from build123d import *

# Parameters (mm, degrees)
SKETCH1_W           = 203.2
SKETCH1_H           = 120.65
BOSS_EXTRUDE1_DEPTH = 50.8
SKETCH2_W           = 196.85
SKETCH2_H           = 114.3
CUT_EXTRUDE1_DEPTH  = 51.8
SKETCH4_W           = 203.2
SKETCH4_H           = 120.65
SKETCH4_W_2         = 196.85
SKETCH4_H_2         = 114.3
BOSS_EXTRUDE2_DEPTH = 6.35
CUT_EXTRUDE5_DEPTH  = 121.65
CUT_EXTRUDE6_REACH  = 205.2
CUT_EXTRUDE7_REACH  = 205.2
SKETCH13_R          = 12.55395
CUT_EXTRUDE8_DEPTH  = 51.8


with BuildPart() as part:
    # Sketch1 → Boss-Extrude1 (new body)
    with BuildSketch(Plane(origin=(0, 0, 0), x_dir=(1, 0, 0), z_dir=(0, 1, 0))):
        Rectangle(SKETCH1_W, SKETCH1_H)
    extrude(amount=BOSS_EXTRUDE1_DEPTH)

    # Sketch2 → Cut-Extrude1 (cut, through all)
    with BuildSketch(Plane(origin=(0, 50.8, 0), x_dir=(1, 0, 0), z_dir=(0, 1, 0))):
        Rectangle(SKETCH2_W, SKETCH2_H)
    extrude(amount=-CUT_EXTRUDE1_DEPTH, mode=Mode.SUBTRACT)

    # Sketch4 → Boss-Extrude2 (add)
    with BuildSketch(Plane(origin=(0, 50.8, 0), x_dir=(1, 0, 0), z_dir=(0, 1, 0))):
        Rectangle(SKETCH4_W, SKETCH4_H)
        Rectangle(SKETCH4_W_2, SKETCH4_H_2, mode=Mode.SUBTRACT)
    extrude(amount=-BOSS_EXTRUDE2_DEPTH)

    # Sketch10 → Cut-Extrude5 (cut, through all)
    with BuildSketch(Plane.XY.offset(60.325)):
        with BuildLine():
            ThreePointArc((-65.9511, 22.225), (-81.206975571, 31.167602912), (-81.556705839, 13.4874))
            Line((-81.556705839, 13.4874), (-70.843294161, 13.4874))
            ThreePointArc((-70.843294161, 13.4874), (-67.257397088, 17.218024429), (-65.9511, 22.225))
        make_face()
        with BuildLine():
            ThreePointArc((-15.1511, 22.225), (-30.406975571, 31.167602912), (-30.756705839, 13.4874))
            Line((-30.756705839, 13.4874), (-20.043294161, 13.4874))
            ThreePointArc((-20.043294161, 13.4874), (-16.457397088, 17.218024429), (-15.1511, 22.225))
        make_face()
        with BuildLine():
            ThreePointArc((35.6489, 22.225), (20.393024429, 31.167602912), (20.043294161, 13.4874))
            Line((20.043294161, 13.4874), (30.756705839, 13.4874))
            ThreePointArc((30.756705839, 13.4874), (34.342602912, 17.218024429), (35.6489, 22.225))
        make_face()
        with BuildLine():
            Line((70.843294161, 13.4874), (81.556705839, 13.4874))
            ThreePointArc((81.556705839, 13.4874), (85.142602912, 17.218024429), (86.4489, 22.225))
            ThreePointArc((86.4489, 22.225), (71.193024429, 31.167602912), (70.843294161, 13.4874))
        make_face()
    extrude(amount=-CUT_EXTRUDE5_DEPTH, mode=Mode.SUBTRACT)

    # Sketch12 → Cut-Extrude6 (cut, up to next)
    with BuildSketch(Plane(origin=(101.6, 0, 0), x_dir=(0, 0, -1), z_dir=(1, 0, 0)), mode=Mode.PRIVATE) as cut_extrude6_sk1:
        with BuildLine():
            ThreePointArc((-16.868294161, 13.4874), (-22.225, 32.4739), (-27.581705839, 13.4874))
            Line((-27.581705839, 13.4874), (-16.868294161, 13.4874))
        make_face()
    cut_extrude6_tool1 = extrude(cut_extrude6_sk1.sketch, amount=-CUT_EXTRUDE6_REACH, mode=Mode.PRIVATE) & part.part
    add(cut_extrude6_tool1.solids().sort_by_distance((101.6, 22.546198, 22.225))[0], mode=Mode.SUBTRACT)
    # Sketch12 → Cut-Extrude6 (cut, up to next)
    with BuildSketch(Plane(origin=(101.6, 0, 0), x_dir=(0, 0, -1), z_dir=(1, 0, 0)), mode=Mode.PRIVATE) as cut_extrude6_sk2:
        with BuildLine():
            ThreePointArc((27.581705839, 13.4874), (22.225, 32.4739), (16.868294161, 13.4874))
            Line((16.868294161, 13.4874), (27.581705839, 13.4874))
        make_face()
    cut_extrude6_tool2 = extrude(cut_extrude6_sk2.sketch, amount=-CUT_EXTRUDE6_REACH, mode=Mode.PRIVATE) & part.part
    add(cut_extrude6_tool2.solids().sort_by_distance((101.6, 22.546198, -22.225))[0], mode=Mode.SUBTRACT)

    # Sketch13 → Cut-Extrude7 (cut, up to next)
    with BuildSketch(Plane.ZY.offset(101.6), mode=Mode.PRIVATE) as cut_extrude7_sk1:
        with Locations((12.7, 28.575)):
            Circle(SKETCH13_R)
    cut_extrude7_tool1 = extrude(cut_extrude7_sk1.sketch, amount=-CUT_EXTRUDE7_REACH, mode=Mode.PRIVATE) & part.part
    add(cut_extrude7_tool1.solids().sort_by_distance((-101.6, 28.575, 12.7))[0], mode=Mode.SUBTRACT)

    # Sketch14 → Cut-Extrude8 (cut, through all)
    with BuildSketch(Plane(origin=(0, 50.8, 0), x_dir=(1, 0, 0), z_dir=(0, 1, 0))):
        Polygon((-98.425, -57.15), (-98.425, -60.325), (101.6, -60.325), (101.6, 60.325), (-98.425, 60.325), align=None)
    extrude(amount=-CUT_EXTRUDE8_DEPTH, mode=Mode.SUBTRACT)


solid = part.part
For this review, take the finished solid that the model builds, in its own axes (mm). Round coordinates to 2 decimals unless told otherwise and drop trailing zeros. Write each loop counter-clockwise with the first axis right and the second up, starting at its lowest first coordinate (ties: lowest second). Pieces come first, ordered by that corner, then holes. Notation, with made-up numbers: M 33.25,32 L 83.25,32 A19 ccw 83.25,67 Z; hole C 2,17.5 d3. An arc over 180 degrees is marked long. Write item = value, one per line. Start each with the question number.
(1) We need section A-A (z = 24). Give the boundary of the cut face in (x, y) (3 decimals), then the cut area to 3 significant figures.
(2) We need section C-C (y = 31.5). Give the boundary of the cut face in (x, z) (3 decimals), then the cut area to 3 significant figures.
(3) We need section B-B (x = -100.55). Give the boundary of the cut face in (y, z) (3 decimals).
(4) For line 1 along Y through (x, z) = (-99.6, 12.7); line 2 along Z through (x, y) = (-99.1, 25) (3 decimals); line 3 along Z through (x, y) = (-100.35, 20) (3 decimals), list the stretches that pass through material, from the lowest coordinate up.
(5) The part is to be moulded in two halves that separate along Y. For faces 1 (the face through (-100, 50.8, -1)), 2 (the face through (-100, 25, -60.325)), 3 (the face through (-100.03, 37.06, 3.45)), say which applies: +Y half, -Y half, draft (parallel to the pull), parting line (faces both ways), or undercut.
Results found:
q1.outline = M -101.6,0 L -98.425,0 L -98.425,23.106 L -101.6,23.106 Z; M -101.6,34.044 L -98.425,34.044 L -98.425,50.8 L -101.6,50.8 Z
q1.area = 127 mm²
q2.outline = M -101.6,-60.325 L -98.425,-60.325 L -98.425,0.492 L -101.6,0.492 Z; M -101.6,24.908 L -98.425,24.908 L -98.425,60.325 L -101.6,60.325 Z
q2.area = 306 mm²
q3.outline = M 0,-60.325 L 50.8,-60.325 L 50.8,60.325 L 0,60.325 Z; hole C 28.575,12.7 d25.108
q4.line_1 = 0 to 16.02, 41.13 to 50.8
q4.line_2 = -60.325 to 0.666, 24.734 to 60.325
q4.line_3 = -60.325 to 3.531, 21.869 to 60.325
q5.face_1 = +Y half
q5.face_2 = draft
q5.face_3 = undercut
